from build123d import *

# Parameters (mm, degrees)
SKETCH1_R           = 2.45
BOSS_EXTRUDE1_DEPTH = 14.6
CHAMFER1_SIZE       = 0.3


with BuildPart() as part:
    # Sketch1 → Boss-Extrude1 (new body)
    with BuildSketch(Plane(origin=(0, 0, 0), x_dir=(1, 0, 0), z_dir=(0, 1, 0))):
        with BuildLine():
            Line((-6, 0), (-6, 10))
            ThreePointArc((-6, 10), (0, 16), (6, 10))
            Line((6, 10), (6, 0))
            ThreePointArc((6, 0), (0, -6), (-6, 0))
        make_face()
        Circle(SKETCH1_R, mode=Mode.SUBTRACT)
        with Locations((0, 10)):
            Circle(SKETCH1_R, mode=Mode.SUBTRACT)
    extrude(amount=BOSS_EXTRUDE1_DEPTH)

    # Chamfer1
    chamfer1_edges = [part.edges().sort_by_distance(p)[0] for p in [
        (-2.45, 0, 0),
        (-2.45, 14.6, 0),
        (0, 14.6, -16),
        (-2.45, 0, -10),
        (-2.45, 14.6, -10),
        (-6, 14.6, -5),
        (0, 14.6, 6),
        (-6, 0, -5),
        (0, 0, -16),
        (6, 0, -5),
        (0, 0, 6),
        (6, 14.6, -5),
    ]]
    chamfer(chamfer1_edges, length=CHAMFER1_SIZE)


solid = part.part
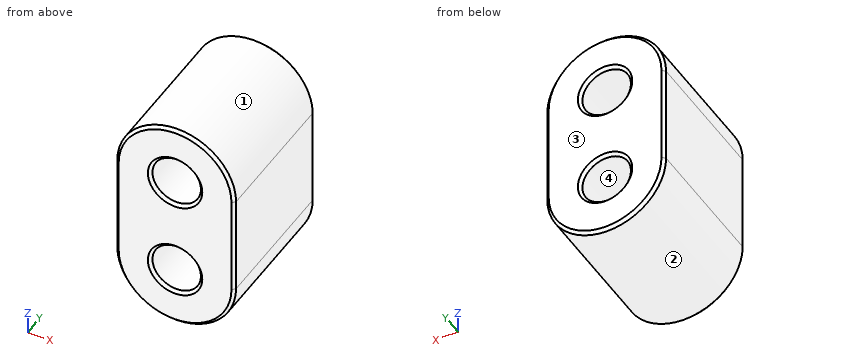
Geometry: final body of the model. Coordinates: model frame, mm. Face numbers are marked on the shaded views. Coordinates: 2 decimals unless noted, no trailing zeros. Order: outer loops, then holes, each group sorted by start corner. A loop starts at its lowest first (then second) coordinate and runs counter-clockwise, first axis right, second up.
(1) Section query A-A (x = 0). Return the cut outline in (y, z), plus the area to 3 significant figures.
(2) Material intervals for probe 1 along Z at (x, y) = (0, 10.5); probe 2 along X at (y, z) = (8.5, 0); probe 3 along X at (y, z) = (8.5, -10.75), sorted ascending.
(3) Section query C-C (x = 2). State how many separate pieces and enclosed holes the cut face has, plus the area to 3 significant figures.
(4) First-contact query: pin 1 (1.5 mm diameter, centred on y = 12.5, z = 1, fed in from +X); pin 2 (6 mm diameter, centred on x = 4, y = 11.5, fed in from +Z); pin 3 (2 mm diameter, centred on x = 3, y = 5.5, fed in from -Z). Flat tips, straight axial feed; report the tip coordinate or a pass-through.
(5) Section query B-B (y = 4.5). Return the cut outline in (x, z).
(6) Draft query along Z for the marked faces 1, 2, 3 and 4. Return one class per face: pulls with the +Z half, pulls with the -Z half, needs draft (parallel to the pull), parting line crosses it, or undercut.
Solution:
1. outline: (0, -15.7) - (0.3, -16) - (14.3, -16) - (14.6, -15.7) - (14.6, -12.75) - (14.3, -12.45) - (0.3, -12.45) - (0, -12.75) - close; (0, -7.25) - (0.3, -7.55) - (14.3, -7.55) - (14.6, -7.25) - (14.6, -2.75) - (14.3, -2.45) - (0.3, -2.45) - (0, -2.75) - close; (0, 2.75) - (0.3, 2.45) - (14.3, 2.45) - (14.6, 2.75) - (14.6, 5.7) - (14.3, 6) - (0.3, 6) - (0, 5.7) - close
1. area: 178 mm2
2. probe 1: z = -16 to -12.45, -7.55 to -2.45, 2.45 to 6
2. probe 2: x = -6 to -2.45, 2.45 to 6
2. probe 3: x = -5.95 to -2.33, 2.33 to 5.95
3. separate pieces: 3
3. enclosed holes: 0
3. area: 228 mm2
4. pin 1: stops at x = 5.99
4. pin 2: stops at z = 5.92
4. pin 3: stops at z = -15.66
5. outline: (-6, -10) arc R6 ccw to (6, -10) - (6, 0) arc R6 ccw to (-6, 0) - close; hole circle Ø4.9 at (0, -10); hole circle Ø4.9 at (0, 0)
6. face 1: pulls with the +Z half
6. face 2: pulls with the -Z half
6. face 3: needs draft
6. face 4: undercut
